Build history of the part. All positions in model axes, mm. Give positions to 0.01 mm unless a question says otherwise; leave off trailing zeros. Order: outer loops, then holes, each group sorted by start corner. A loop starts at its lowest first (then second) coordinate and runs counter-clockwise, first axis right, second up. Notation, with made-up numbers: (39, 62) -> (98, 62) arc R17 ccw to (98, 68) -> close; hole circle Ø11 at (87.5, 13). An arc over 180 degrees is marked (long way). One line per item, written item: value. Start each with the question number.
(1) Two-plate mould, pull along X, no slides. Class faces 1 (the cylindrical face through (-0.29, -2.49, 2.23)), 2 (the flat face through (7.6, -2.9, 5.4)), 3 (the cylindrical face through (-6, -2, 0)): +X half, -X half, draft (parallel to the pull), parting line (faces both ways), or undercut.
(2) Saw through at B-B on y = -1.75. Give the cut face in (x, z).
(3) Saw through at A-A on z = 0. Give the cut face in (x, y).
(4) Saw through at C-C on x = 5.75. Give the cut face in (y, z), plus the area to 3 significant figures.
(5) Saw through at D-D on y = -3.15. Give the cut face in (x, z), plus the area to 3 significant figures.
(6) Probe line 1 (Z direction, x = 0, y = -2); line 2 (X direction, y = -1.8, z = 0.25); line 3 (X direction, y = -2.55, z = 0). List the from-to ranges inside material, lowest first.
```python
from build123d import *

# Parameters (mm, degrees)
PAD001_DEPTH    = 2
CHAMFER001_SIZE = 1.2
SKETCH005_R     = 2.25
HOLE001_DEPTH   = 25


with BuildPart() as part:
    # Sketch004 → Pad001 (new body)
    with BuildSketch(Plane.XZ):
        with BuildLine():
            ThreePointArc((0, 6), (-6, 0), (0, -6))
            Line((0, -6), (15, -6))
            ThreePointArc((15, -6), (21, 0), (15, 6))
            Line((15, 6), (0, 6))
        make_face()
    extrude(amount=PAD001_DEPTH)

    # Chamfer001
    chamfer001_edges = [part.edges().sort_by_distance(p)[0] for p in [
        (7.5, -2, 6),
    ]]
    chamfer(chamfer001_edges, length=CHAMFER001_SIZE)

    # Sketch005 → Hole001 (cut)
    with BuildSketch(Plane.XZ):
        Circle(SKETCH005_R)
        with Locations((15, 0)):
            Circle(SKETCH005_R)
    extrude(amount=HOLE001_DEPTH, mode=Mode.SUBTRACT)


with BuildPart() as part_1:
    # Body001 placement: moved
    add(part.part.moved(Location((0, -1.5, 0))))


solid = part_1.part
```
Results below:
1. face 1: undercut
1. face 2: draft
1. face 3: -X half
2. outline: (0, -6) -> (15, -6) arc R6 ccw to (15, 6) -> (0, 6) arc R6 ccw to start; hole circle Ø4.5 at (0, 0); hole circle Ø4.5 at (15, 0)
3. outline: (-6, -2.3) -> (-4.8, -3.5) -> (-2.25, -3.5) -> (-2.25, -1.5) -> (-6, -1.5) -> close; (2.25, -3.5) -> (12.75, -3.5) -> (12.75, -1.5) -> (2.25, -1.5) -> close; (17.25, -3.5) -> (19.8, -3.5) -> (21, -2.3) -> (21, -1.5) -> (17.25, -1.5) -> close
4. outline: (-3.5, -4.8) -> (-2.3, -6) -> (-1.5, -6) -> (-1.5, 6) -> (-2.3, 6) -> (-3.5, 4.8) -> close
4. area: 22.6 mm²
5. outline: (0, -5.15) -> (15, -5.15) arc R5.15 ccw to (15, 5.15) -> (0, 5.15) arc R5.15 ccw to start; hole circle Ø4.5 at (0, 0); hole circle Ø4.5 at (15, 0)
5. area: 206 mm²
6. line 1: z = -6 to -2.25, 2.25 to 6
6. line 2: x = -5.99 to -2.24, 2.24 to 12.76, 17.24 to 20.99
6. line 3: x = -5.75 to -2.25, 2.25 to 12.75, 17.25 to 20.75
